Geometry check sheet. Reference: the model listing, model coordinates, mm. A direction names the side the tool comes from. Give positions to 0.01 mm unless a question says otherwise; leave off trailing zeros. Write each loop counter-clockwise with the first axis right and the second up, starting at its lowest first coordinate (ties: lowest second). Pieces come first, ordered by that corner, then holes. Notation, with made-up numbers: (76, -31) -> (95, -31) arc R17 cw to (95, 0) -> close; hole circle Ø9 at (32.5, 72). An arc over 180 degrees is marked (long way). One line per item, written item: value.
from build123d import *

# Parameters (mm, degrees)
BOSS_EXTRUDE3_DEPTH      = 19.844397107
BOSS_EXTRUDE3_DEPTH_BACK = 1
SKETCH4_R                = 84.5
BOSS_EXTRUDE4_DEPTH      = 100
SKETCH6_R                = 84.5
BOSS_EXTRUDE6_DEPTH      = 100
BOSS_EXTRUDE7_DEPTH      = 20


with BuildPart() as part:
    # Sketch3 → Boss-Extrude3 (new, two sides: drawn at the far end of the back side and taken through both)
    with BuildSketch(Plane(origin=(0, 0, 0), x_dir=(1, 0, 0), z_dir=(0, 1, 0)).offset(-BOSS_EXTRUDE3_DEPTH_BACK)):
        with BuildLine():
            ThreePointArc((-84.5, 140.346835397), (0, 55.846835397), (84.5, 140.346835397))
            Line((84.5, 140.346835397), (-84.5, 140.346835397))
        make_face()
        with BuildLine():
            Line((-84.5, 140.346835397), (84.5, 140.346835397))
            ThreePointArc((84.5, 140.346835397), (0, 224.846835397), (-84.5, 140.346835397))
        make_face()
        with BuildLine():
            ThreePointArc((-84.5, 140.346835397), (0, 224.846835397), (84.5, 140.346835397))
            Line((84.5, 140.346835397), (84.5, 840.346835397))
            ThreePointArc((84.5, 840.346835397), (0, 755.846835397), (-84.5, 840.346835397))
            Line((-84.5, 840.346835397), (-84.5, 140.346835397))
        make_face()
        with BuildLine():
            ThreePointArc((-84.5, 840.346835397), (0, 755.846835397), (84.5, 840.346835397))
            Line((84.5, 840.346835397), (-84.5, 840.346835397))
        make_face()
        with BuildLine():
            Line((-84.5, 840.346835397), (84.5, 840.346835397))
            ThreePointArc((84.5, 840.346835397), (0, 924.846835397), (-84.5, 840.346835397))
        make_face()
    extrude(amount=BOSS_EXTRUDE3_DEPTH + BOSS_EXTRUDE3_DEPTH_BACK)

    # Sketch4 → Boss-Extrude4 (add)
    with BuildSketch(Plane(origin=(0, 19.844397107, 0), x_dir=(1, 0, 0), z_dir=(0, 1, 0))):
        with Locations(Location((0, 140.346835397, 0), (0, 0, 270))):
            Circle(SKETCH4_R)
    extrude(amount=BOSS_EXTRUDE4_DEPTH)

    # Sketch6 → Boss-Extrude6 (add)
    with BuildSketch(Plane(origin=(0, 19.844397107, 0), x_dir=(1, 0, 0), z_dir=(0, 1, 0))):
        with Locations(Location((0, 840.346835397, 0), (0, 0, 270))):
            Circle(SKETCH6_R)
    extrude(amount=BOSS_EXTRUDE6_DEPTH)

    # Sketch7 → Boss-Extrude7 (add)
    with BuildSketch(Plane(origin=(0, 119.844397107, 0), x_dir=(1, 0, 0), z_dir=(0, 1, 0))):
        with BuildLine():
            ThreePointArc((-84.5, 140.346835397), (0, 55.846835397), (84.5, 140.346835397))
            Line((84.5, 140.346835397), (-84.5, 140.346835397))
        make_face()
        with BuildLine():
            Line((-84.5, 140.346835397), (84.5, 140.346835397))
            ThreePointArc((84.5, 140.346835397), (0, 224.846835397), (-84.5, 140.346835397))
        make_face()
        with BuildLine():
            ThreePointArc((-84.5, 140.346835397), (0, 224.846835397), (84.5, 140.346835397))
            Line((84.5, 140.346835397), (84.5, 840.32890922))
            ThreePointArc((84.5, 840.32890922), (0, 755.82890922), (-84.5, 840.32890922))
            Line((-84.5, 840.32890922), (-84.5, 140.346835397))
        make_face()
        with BuildLine():
            ThreePointArc((-84.5, 840.32890922), (0, 755.82890922), (84.5, 840.32890922))
            Line((84.5, 840.32890922), (-84.5, 840.32890922))
        make_face()
        with BuildLine():
            Line((-84.5, 840.32890922), (84.5, 840.32890922))
            ThreePointArc((84.5, 840.32890922), (0, 924.82890922), (-84.5, 840.32890922))
        make_face()
    extrude(amount=BOSS_EXTRUDE7_DEPTH)


solid = part.part
1) Scan lines: probe 1 along Z at (x, y) = (-1, 37); probe 2 along Y at (x, z) = (-54, -764); probe 3 along Z at (x, y) = (47.5, 76). Record each from-to range of solid material in increasing order.
Verdict:
probe 1: -924.84 to -755.85, -224.84 to -55.85
probe 2: -1 to 19.84, 119.84 to 139.84
probe 3: -910.23 to -770.46, -210.23 to -70.46
2) Tool access check on faces 1 (the cylindrical face through (3.715, 58.576, -924.765)), 2 (the flat face through (-84.5, 130, -495)). Record the directions out of +Z, -Z, +X, -X, +Y, -Y that give a thin tool (end or side, any length) a straight path to the whole face; none if there is none.
Verdict:
face 1: none
face 2: +Z, -Z, -X, +Y, -Y
3) Depth check by flat-ended pin: pin 1 Ø2 at (x, y) = (4.5, 59.5) entering from -Z; pin 2 Ø5 at (x, y) = (-8.5, 96.5) entering from +Z. Enter the tip coordinate at first touch or a pass-through.
Verdict:
pin 1: z = -924.77
pin 2: z = -56.06
4) Sectioned sample at A-A on z = -632. Record the cut outline in (x, y), plus the area to 3 significant figures.
Verdict:
outline: (-84.5, -1) -> (84.5, -1) -> (84.5, 19.84) -> (-84.5, 19.84) -> close; (-84.5, 119.84) -> (84.5, 119.84) -> (84.5, 139.84) -> (-84.5, 139.84) -> close
area: 6,900 mm^2
5) Mould release check, pull along Y, two halves, no side actions. Record for faces 3 (the cylindrical face through (31.449, 68.436, -61.917)), 4 (the flat face through (-1, -1, -496)), 5 (the flat face through (-84.5, 9, -495)), 6 (the flat face through (-1, 139.844, -496)): released by +Y, released by -Y, zero draft, split by the parting line, or undercut.
Verdict:
face 3: undercut
face 4: released by -Y
face 5: zero draft
face 6: released by +Y
6) Sectioned sample at C-C on y = 108. Record the cut outline in (x, z), plus the area to 3 significant figures.
Verdict:
outline: circle Ø169 at (0, -840.35); circle Ø169 at (0, -140.35)
area: 44,900 mm^2
